The drawing under review shows one solid part. Ordinate dimensions are in mm from its lowest x, y, z. Round coordinates to 2 decimals unless told otherwise and drop trailing zeros. Order: outer loops, then holes, each group sorted by start corner. A loop starts at its lowest first (then second) coordinate and runs counter-clockwise, first axis right, second up. Notation, with made-up numbers: M 22.25,32 L 73.25,32 A35 cw 73.25,64 Z; hole C -19.5,-10.75 d1. An arc over 180 degrees is marked long. Answer as a JSON object with one key per item and string values. Group by question number.
1. Add section A-A on y = 30. State the section outline as (x, z) points, and give its area (3 significant figures).
2. Clearance check with flat-ended pins moving along their axes: P1, Ø1.5, axis at y = 19.5, z = 14, coming from the -X side; P2, Ø17, axis at x = 641.5, z = 24, coming from the +Y side; P3, Ø7.5, axis at x = 29, y = 24, coming from the -Z side; P4, Ø1, axis at x = 167, y = 19, coming from the -Z side. State where each tip first meets the part, or that it passes through.
3. Add section B-B on z = 12. State the section outline as (x, y) points.
4. To check wall thickness, follow probe 1 along X at (y, z) = (34.5, 41.5); probe 2 along Y at (x, z) = (28.5, 20); probe 3 along Z at (x, y) = (36, 28). State the ranges of each line that lie inside material, in increasing order. Write a range as [from, to].
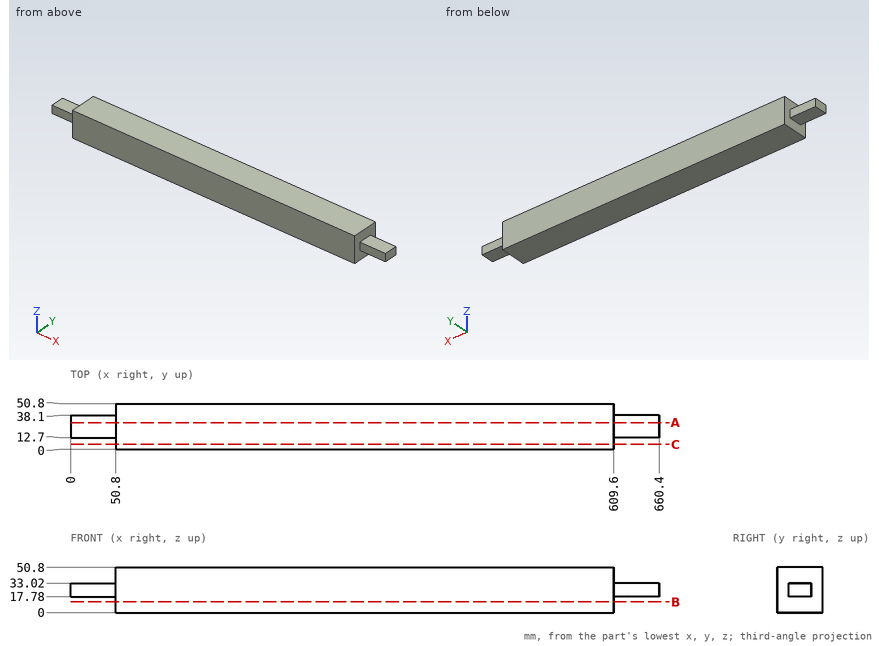
Recorded:
{
 "1": {"outline": "M 0,17.78 L 50.8,17.78 L 50.8,0 L 609.6,0 L 609.6,17.78 L 660.4,17.78 L 660.4,33.02 L 609.6,33.02 L 609.6,50.8 L 50.8,50.8 L 50.8,33.02 L 0,33.02 Z", "area": "29,900 mm²"},
 "2": {"P1": "stops at x = 50.8", "P2": "stops at y = 38.1", "P3": "stops at z = 17.78", "P4": "stops at z = 0"},
 "3": {"outline": "M 50.8,0 L 609.6,0 L 609.6,50.8 L 50.8,50.8 Z"},
 "4": {"probe 1": "x = [50.8, 609.6]", "probe 2": "y = [12.7, 38.1]", "probe 3": "z = [17.78, 33.02]"}
}
